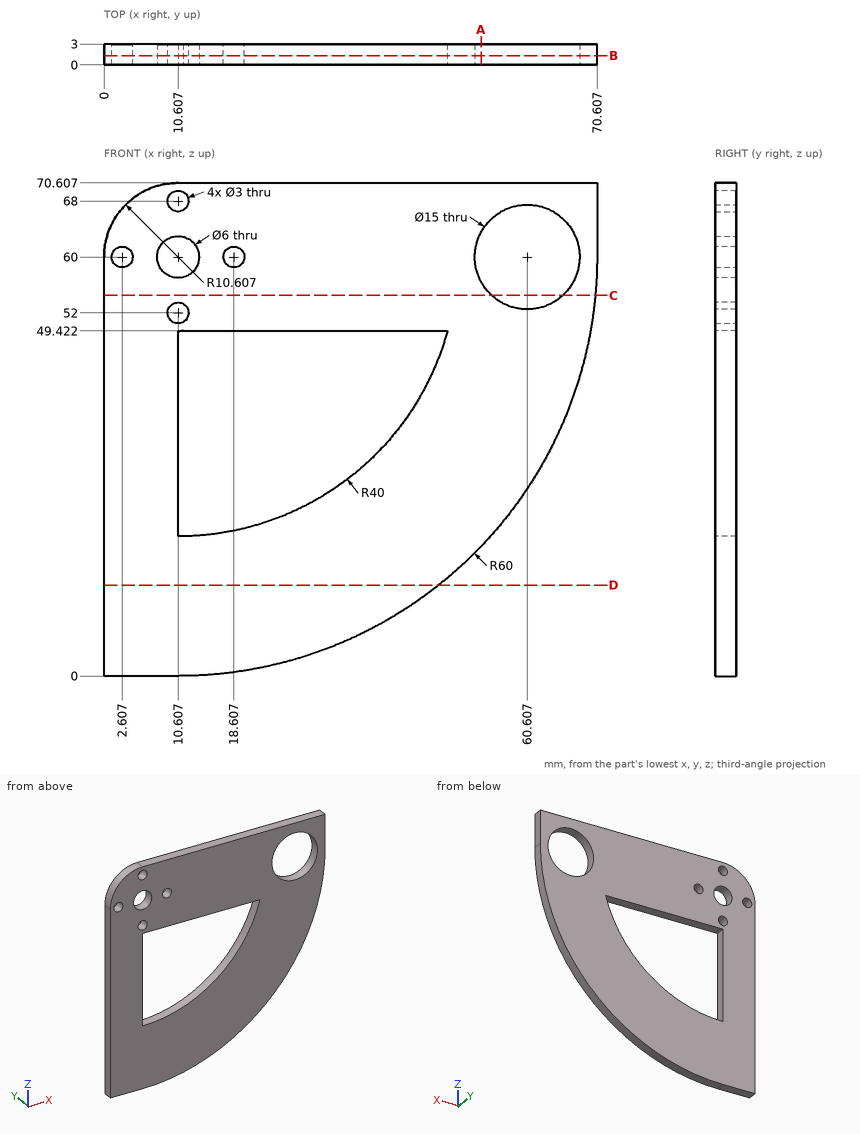
Part print with two shaded views. Sizes in mm from the minimum x, y, z corner. Coordinates: 2 decimals unless noted, no trailing zeros. Write each loop counter-clockwise with the first axis right and the second up, starting at its lowest first coordinate (ties: lowest second). Pieces come first, ordered by that corner, then holes. Notation, with made-up numbers: (-10.5, -33) - (20.5, -33) arc R18 ccw to (20.5, 0) - close; hole circle Ø10 at (-17.75, 21.25). An arc over 180 degrees is marked (long way). Use a Markdown table: item, result. Add a question column.
Item 1: Band-saw the part on C-C, the plane z = 54.5. Write the cut outline in (x, y) (1 decimal).
Item 2: Band-saw the part on A-A, the plane x = 54. Write the cut outline in (y, z), and give its area (3 significant figures).
Item 3: Drill centre lines: line 1 along X through (y, z) = (1.9, 60); line 2 along Z through (x, y) = (18, 0.5); line 3 along X through (y, z) = (0.45, 34) (1 decimal). Where is each one in solid material? Low to high.
Item 4: Drop a flat-ended pin along its axis: pin 1 (1.5 mm diameter, centred on x = 47, y = 1, fed in from -Z) (1 decimal). Give the stop position or say it passes through.
Item 5: Band-saw the part on D-D, the plane z = 13. Write the cut outline in (x, y).
Item 6: Band-saw the part on B-B, the plane y = 1.35. Write the cut outline in (x, z).
A:
| question | item | result |
|---|---|---|
| 1 | outline | (0, 0) - (55.5, 0) - (55.5, 3) - (0, 3) - close; (65.7, 0) - (70.4, 0) - (70.4, 3) - (65.7, 3) - close |
| 2 | outline | (0, 18.56) - (3, 18.56) - (3, 56.45) - (0, 56.45) - close; (0, 63.55) - (3, 63.55) - (3, 70.61) - (0, 70.61) - close |
| 2 | area | 135 mm² |
| 3 | line 1 | x = 0 to 1.11, 4.11 to 7.61, 13.61 to 17.11, 20.11 to 53.11, 68.11 to 70.61 |
| 3 | line 2 | z = 0.46 to 20.69, 49.42 to 58.63, 61.37 to 70.61 |
| 3 | line 3 | x = 0 to 10.6, 41 to 64.7 |
| 4 | pin 1 | stops at z = 11.7 |
| 5 | outline | (0, 0) - (47.9, 0) - (47.9, 3) - (0, 3) - close |
| 6 | outline | (0, 0) - (10.61, 0) arc R60 ccw to (70.61, 60) - (70.61, 70.61) - (10.61, 70.61) arc R10.61 ccw to (0, 60) - close; hole circle Ø3 at (2.61, 60); hole circle Ø6 at (10.61, 60); hole circle Ø3 at (10.61, 52); hole circle Ø3 at (10.61, 68); hole (10.61, 20) arc R40 ccw to (49.18, 49.42) - (11.38, 49.42) arc R10.61 cw to (10.61, 49.39) - close; hole circle Ø3 at (18.61, 60); hole circle Ø15 at (60.61, 60) |
